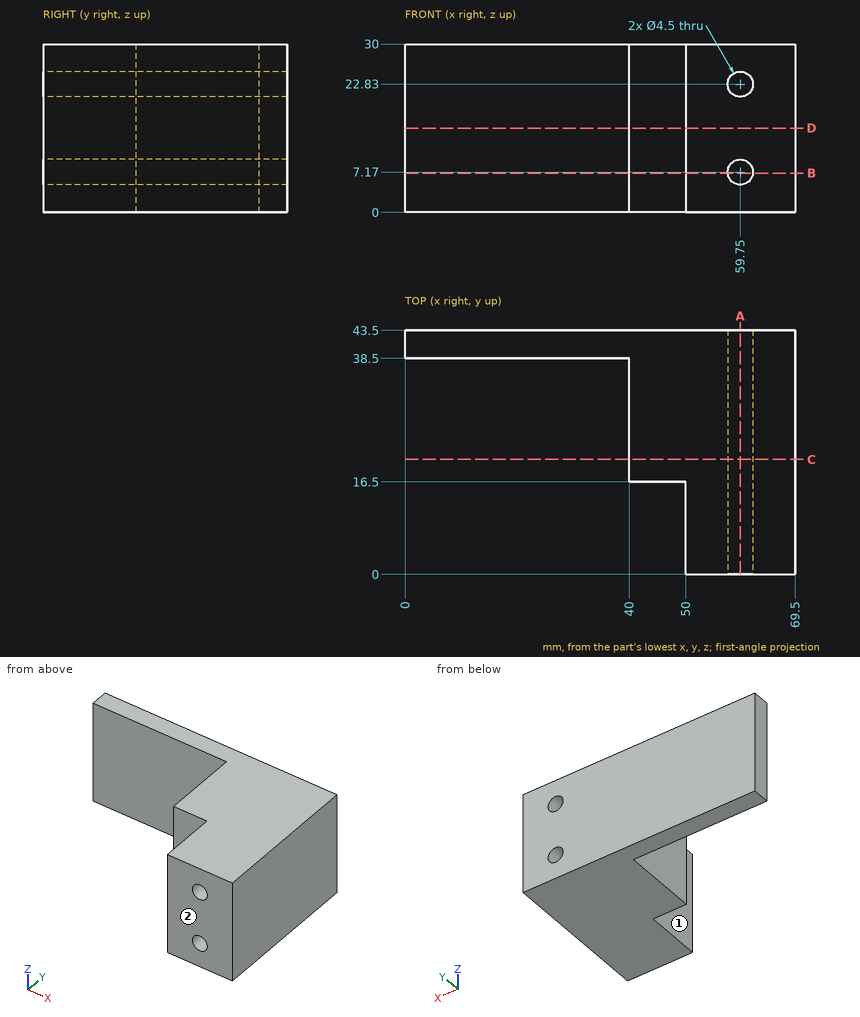
Answer from the drawing. Dimensions are ordinates in mm from the lowest x, y and z of the part. A direction names the side the tool comes from. Round coordinates to 2 decimals unless told otherwise and drop trailing zeros. Write each loop counter-clockwise with the first axis right and the second up, starting at its lowest first coordinate (ties: lowest second). Pieces come first, ordered by that corner, then holes. Notation, with made-up numbers: (79, 17.5) - (104, 17.5) arc R12 ccw to (104, 37.5) - close; hole circle Ø5 at (-3, 46.25). An arc over 180 degrees is marked (long way). Use a Markdown table: item, result.
(1) Each of these flat-tipped pins is pushed along its axis until it touches: pin 1 Ø5 at (x, z) = (46.5, 18) entering from -Y; pin 2 Ø11 at (y, z) = (23, 9.5) entering from -X; pin 3 Ø15 at (x, z) = (21, 8.5) entering from -Y; pin 4 Ø4 at (x, z) = (59.75, 7.17) entering from +Y. Where does it stop, or does it pass through?
Reported:
| item | result |
|---|---|
| pin 1 | y = 16.5 |
| pin 2 | x = 40 |
| pin 3 | y = 38.5 |
| pin 4 | through |
(2) The part is cut by section D-D (z = 15). Write down the section's boundary in (x, y), then the cut area to 3 significant figures.
Reported:
| item | result |
|---|---|
| outline | (0, 38.5) - (40, 38.5) - (40, 16.5) - (50, 16.5) - (50, 0) - (69.5, 0) - (69.5, 43.5) - (0, 43.5) - close |
| area | 1,320 mm2 |
(3) Straight lines are drawn through the part: line 1 along X through (y, z) = (33.5, 7); line 2 along Y through (x, z) = (35, 3.5); line 3 along X through (y, z) = (34, 28). For each, find the intervals that lie inside material, in ascending order. Write a range as [from, to].
Reported:
| item | result |
|---|---|
| line 1 | [40, 57.51], [61.99, 69.5] |
| line 2 | [38.5, 43.5] |
| line 3 | [40, 69.5] |
(4) The part is cut by section A-A (x = 59.75). Write down the section's boundary in (y, z).
Reported:
| item | result |
|---|---|
| outline | (0, 0) - (43.5, 0) - (43.5, 4.92) - (0, 4.92) - close; (0, 9.42) - (43.5, 9.42) - (43.5, 20.58) - (0, 20.58) - close; (0, 25.08) - (43.5, 25.08) - (43.5, 30) - (0, 30) - close |
(5) Which of the six approach directions +Z, -Z, +X, -X, +Y, -Y give full straight-line access (tool end or side, diameter ignored) to the marked faces 1 and 2?
Reported:
| item | result |
|---|---|
| face 1 | +Z, -Z, -X, -Y |
| face 2 | +Z, -Z, +X, -X, -Y |
(6) The part is cut by section B-B (z = 7). Write down the section's boundary in (x, y).
Reported:
| item | result |
|---|---|
| outline | (0, 38.5) - (40, 38.5) - (40, 16.5) - (50, 16.5) - (50, 0) - (57.51, 0) - (57.51, 43.5) - (0, 43.5) - close; (61.99, 0) - (69.5, 0) - (69.5, 43.5) - (61.99, 43.5) - close |
(7) The part is cut by section C-C (y = 20.5). Write down the section's boundary in (x, z), then the cut area to 3 significant figures.
Reported:
| item | result |
|---|---|
| outline | (40, 0) - (69.5, 0) - (69.5, 30) - (40, 30) - close; hole circle Ø4.5 at (59.75, 7.17); hole circle Ø4.5 at (59.75, 22.83) |
| area | 853 mm2 |
